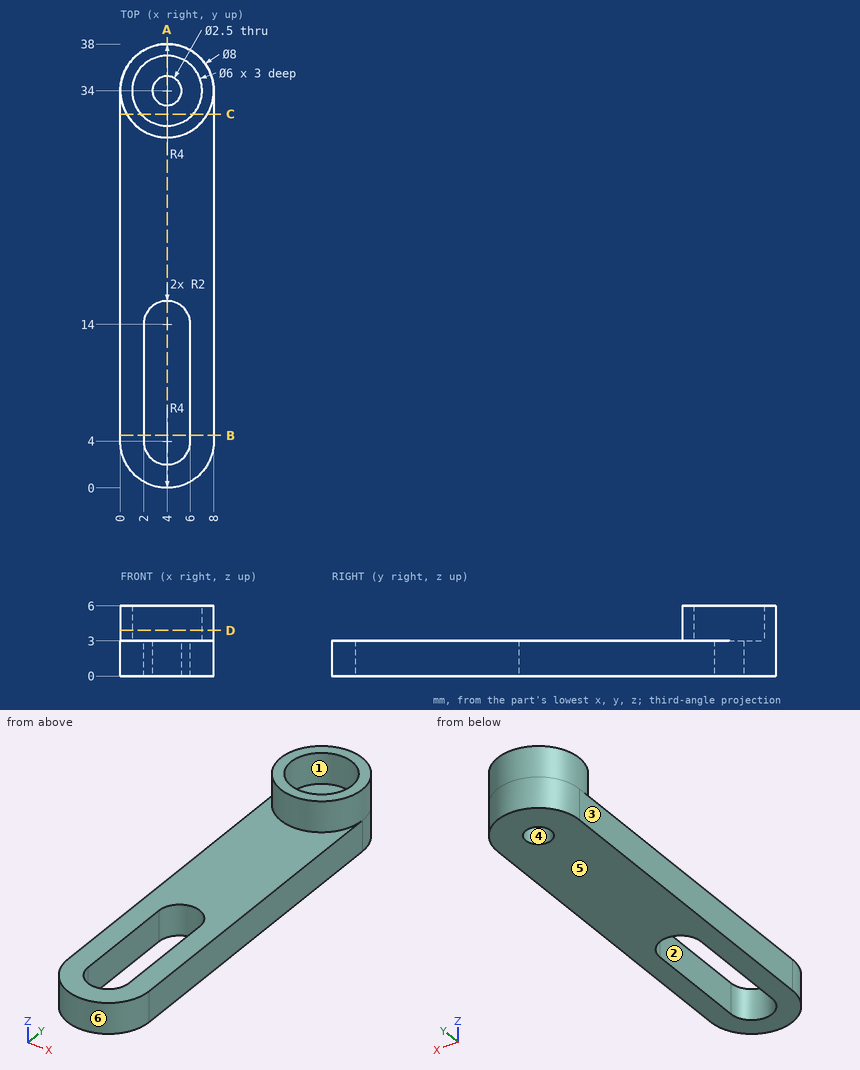
Source: three-view drawing plus pictorial views. Frame: mm from the lowest corner of the part. A direction names the side the tool comes from. Give positions to 0.01 mm unless a question says otherwise; leave off trailing zeros. Order: outer loops, then holes, each group sorted by start corner. A loop starts at its lowest first (then second) coordinate and runs counter-clockwise, first axis right, second up. Notation, with made-up numbers: (51.5, -0.75) -> (58.5, -0.75) arc R17 ccw to (58.5, 20.25) -> close; hole circle Ø9 at (85.5, 17.25). An arc over 180 degrees is marked (long way). Write each question's results on one line, items separated by ' | '. Start each with the question number.
Item 1: Set-up query: the marked faces 1, 2 and 3. Return all of +Z, -Z, +X, -X, +Y, -Y with unobstructed straight access to the full face (end or side cutting, diameter ignored); none if empty.
Item 2: Mould query, pull axis Y, two halves, no side actions, for the marked faces 4, 5 and 6. Classes: pulls with the +Y half, pulls with the -Y half, needs draft (parallel to the pull), parting line crosses it, or undercut.
Item 3: Cut plane D-D on z = 3.9. Return the cut outline in (x, y).
Item 4: Cut plane A-A on x = 4. Return the cut outline in (y, z), then the cut area to 3 significant figures.
Item 5: Cut plane C-C on y = 32. Return the cut outline in (x, z).
Item 6: Cut plane B-B on y = 4.5. Return the cut outline in (x, z), then the cut area to 3 significant figures.
Item 7: Contact query for flat-ended pins moving along their axis: P1, Ø2, axis at y = 13, z = 4.5, coming from the +X side; P2, Ø4, axis at x = 4, y = 34, coming from the +Z side. Output: stop coordinate, or through.
Item 8: Line query: line 1 (Y direction, x = 4, z = 0.85); line 2 (X direction, y = 34, z = 2); line 3 (X direction, y = 6, z = 2.25). Output: solid intervals per line, ascending.
Established:
1) face 1: +Z | face 2: +Z, -Z | face 3: +Z, -Z, -X, +Y, -Y
2) face 4: undercut | face 5: needs draft | face 6: pulls with the -Y half
3) outline: circle Ø8 at (4, 34); hole circle Ø6 at (4, 34)
4) outline: (0, 0) -> (2, 0) -> (2, 3) -> (0, 3) -> close; (16, 0) -> (32.75, 0) -> (32.75, 3) -> (31, 3) -> (31, 6) -> (30, 6) -> (30, 3) -> (16, 3) -> close; (35.25, 0) -> (38, 0) -> (38, 6) -> (37, 6) -> (37, 3) -> (35.25, 3) -> close | area: 70.5 mm^2
5) outline: (0, 0) -> (8, 0) -> (8, 3) -> (7.46, 3) -> (7.46, 6) -> (6.24, 6) -> (6.24, 3) -> (1.76, 3) -> (1.76, 6) -> (0.54, 6) -> (0.54, 3) -> (0, 3) -> close
6) outline: (0, 0) -> (2, 0) -> (2, 3) -> (0, 3) -> close; (6, 0) -> (8, 0) -> (8, 3) -> (6, 3) -> close | area: 12.0 mm^2
7) P1: through | P2: z = 3
8) line 1: 0 to 2, 16 to 32.75, 35.25 to 38 | line 2: 0 to 2.75, 5.25 to 8 | line 3: 0 to 2, 6 to 8
